Work out the finished part from the listing and answer in its coordinate system (mm). Round coordinates to 2 decimals unless told otherwise and drop trailing zeros. Order: outer loops, then holes, each group sorted by start corner. A loop starts at its lowest first (then second) coordinate and runs counter-clockwise, first axis right, second up. Notation, with made-up numbers: (61.5, -38.5) - (108.5, -38.5) arc R23 cw to (108.5, -1.5) - close; hole circle Ø2 at (-38.75, -10). An arc over 180 degrees is marked (long way). One line per question, with ' | ' between items. Start each with the question number.
from build123d import *

# Parameters (mm, degrees)
SKETCH1_R                     = 10
BOSS_EXTRUDE1_DEPTH           = 3
CSK_FOR_M4_SFHCS1_D           = 4.5
CSK_FOR_M4_SFHCS1_DEPTH       = 5.1
CSK_FOR_M4_SFHCS1_CSINK_D     = 8.96
CSK_FOR_M4_SFHCS1_CSINK_ANGLE = 90
CSK_FOR_M4_SFHCS1_TIP         = 1.351936393


with BuildPart() as part:
    # Sketch1 → Boss-Extrude1 (new body)
    with BuildSketch(Plane.XY):
        with BuildLine():
            Line((-21.398771617, 2.935661447), (-15.586431393, -14.952882373))
            ThreePointArc((-15.586431393, -14.952882373), (-13.225168177, -18.202882373), (-9.404564037, -19.44427191))
            Line((-9.404564037, -19.44427191), (9.404564037, -19.44427191))
            ThreePointArc((9.404564037, -19.44427191), (13.225168177, -18.202882373), (15.586431393, -14.952882373))
            Line((15.586431393, -14.952882373), (21.398771617, 2.935661447))
            ThreePointArc((21.398771617, 2.935661447), (21.398771617, 6.952882373), (19.037508401, 10.202882373))
            Line((19.037508401, 10.202882373), (3.82060414, 21.258610463))
            ThreePointArc((3.82060414, 21.258610463), (0, 22.5), (-3.82060414, 21.258610463))
            Line((-3.82060414, 21.258610463), (-19.037508401, 10.202882373))
            ThreePointArc((-19.037508401, 10.202882373), (-21.398771617, 6.952882373), (-21.398771617, 2.935661447))
        make_face()
        Circle(SKETCH1_R, mode=Mode.SUBTRACT)
    extrude(amount=-BOSS_EXTRUDE1_DEPTH)

    # CSK for M4 SFHCS1
    with Locations(Plane.XY):
        with Locations((0, 16), (15.216904261, 4.94427191), (9.404564037, -12.94427191), (-9.404564037, -12.94427191), (-15.216904261, 4.94427191)):
            CounterSinkHole(CSK_FOR_M4_SFHCS1_D / 2, CSK_FOR_M4_SFHCS1_CSINK_D / 2, depth=CSK_FOR_M4_SFHCS1_DEPTH, counter_sink_angle=CSK_FOR_M4_SFHCS1_CSINK_ANGLE)
            with Locations((0, 0, -(CSK_FOR_M4_SFHCS1_DEPTH + CSK_FOR_M4_SFHCS1_TIP / 2))):  # 118° drill point
                Cone(0, CSK_FOR_M4_SFHCS1_D / 2, CSK_FOR_M4_SFHCS1_TIP, mode=Mode.SUBTRACT)


solid = part.part
1) Straight lines are drawn through the part: line 1 (Y direction, x = 7, z = -0.8); line 2 (X direction, y = -14, z = -2.8); line 3 (X direction, y = 6, z = -1.6). For each, find the intervals that lie inside material, in ascending order.
2) Determine the mould class of faces 1 (the cylindrical face through (11.06, -11.42, -2.62)), 2 (the flat face through (11.54, 15.65, -1.48)), 3 (the flat face through (18.452, -6.134, -1.479)), 4 (the flat face through (-10, 2, 0)) for opening direction Y: released by +Y, released by -Y, zero draft, split by the parting line, or undercut.
3) Section C-C on x = 8 is taken. Give the number of separate pieces and of enclosed holes in the cut face, and give its area (3 significant figures).
4) Flat-ended cylindrical pins translate along their axes: pin 1 (1 mm diameter, centred on x = 14, y = 1.5, fed in from +Z); pin 2 (5 mm diameter, centred on x = 0, y = 16, fed in from +Z); pin 3 (4 mm diameter, centred on x = 9.4, y = -12.94, fed in from +Z); pin 4 (7 mm diameter, centred on x = -9.4, y = -12.94, fed in from +Z). Find the tip coordinate at first contact, or state that the pin passes through.
5) Section A-A on x = 0 is taken. Give the vertices of the cut face in (y, z).
6) Section B-B on y = 16 is taken. Give the vertices of the cut face in (x, z), and give its area (3 significant figures).
Recorded:
1) line 1: y = -19.44 to -15.73, -10.16 to -7.14, 7.14 to 18.95 | line 2: x = -15.9 to -11.39, -7.42 to 7.42, 11.39 to 15.9 | line 3: x = -21.63 to -17.9, -12.54 to -8, 8 to 12.54, 17.9 to 21.63
2) face 1: undercut | face 2: released by +Y | face 3: released by -Y | face 4: zero draft
3) separate pieces: 3 | enclosed holes: 0 | area: 60.7 mm²
4) pin 1: stops at z = -0.33 | pin 2: stops at z = -1.98 | pin 3: passes through | pin 4: stops at z = -0.97
5) outline: (-19.44, -3) - (-10, -3) - (-10, 0) - (-19.44, 0) - close; (10, -3) - (13.75, -3) - (13.75, -2.23) - (11.52, 0) - (10, 0) - close; (18.25, -3) - (22.5, -3) - (22.5, 0) - (20.48, 0) - (18.25, -2.23) - close
6) outline: (-11.06, -3) - (-2.25, -3) - (-2.25, -2.23) - (-4.48, 0) - (-11.06, 0) - close; (2.25, -3) - (11.06, -3) - (11.06, 0) - (4.48, 0) - (2.25, -2.23) - close | area: 47.9 mm²
